```python
from build123d import *

# Parameters (mm, degrees)
SKETCH1_R           = 11.75
BOSS_EXTRUDE1_DEPTH = 60
CUT_EXTRUDE1_DEPTH  = 63.258533552
CUT_EXTRUDE2_DEPTH  = 64.608686514


with BuildPart() as part:
    # Sketch1 → Boss-Extrude1 (new body)
    with BuildSketch(Plane(origin=(0, 0, 0), x_dir=(0, 0, -1), z_dir=(1, 0, 0))):
        Circle(SKETCH1_R)
    extrude(amount=BOSS_EXTRUDE1_DEPTH)

    # Sketch2 → Cut-Extrude1 (cut, through all)
    with BuildSketch(Plane.ZY):
        with BuildLine():
            Line((5.8, 10.218732798), (5.8, -10.218732798))
            ThreePointArc((5.8, -10.218732798), (11.75, 0), (5.8, 10.218732798))
        make_face()
    extrude(amount=-CUT_EXTRUDE1_DEPTH, mode=Mode.SUBTRACT)

    # Sketch3 → Cut-Extrude2 (cut, through all)
    with BuildSketch(Plane.XY.offset(5.8)):
        with BuildLine():
            Line((0, 11.75), (60, 11.75))
            Line((60, 11.75), (60, -11.75))
            Line((60, -11.75), (44.282856857, -11.75))
            ThreePointArc((44.282856857, -11.75), (30, -5.75), (15.717143143, -11.75))
            Line((15.717143143, -11.75), (0, -11.75))
            Line((0, -11.75), (0, 11.75))
        make_face()
    extrude(amount=-CUT_EXTRUDE2_DEPTH, mode=Mode.SUBTRACT)


solid = part.part
```
Check sheet for the modelled part. Datum: model origin and axes. Units: mm. Give positions to 0.01 mm unless a question says otherwise; leave off trailing zeros. Order: outer loops, then holes, each group sorted by start corner. A loop starts at its lowest first (then second) coordinate and runs counter-clockwise, first axis right, second up. Notation, with made-up numbers: M 43,39 L 99,39 A21 ccw 99,71 Z; hole C -32,-16.75 d8. An arc over 180 degrees is marked long. Answer in a Markdown table with one row per item.
1) Cross-section at B-B, the plane z = 1.5. Enter the section's corners in (x, y), plus the area to 3 significant figures.
Filled sheet:
| item | result |
|---|---|
| outline | M 15.81,-11.65 L 44.19,-11.65 A20 ccw Z |
| area | 115 mm2 |
2) Gauge pin test, flat ends, axial feed: P1, Ø1, axis at x = 26, z = -6, coming from the +Y side; P2, Ø1.5, axis at x = 40.5, z = -5.5, coming from the -Y side; P3, Ø3, axis at y = -7.5, z = -3, coming from the -X side. Record the tip position at first contact, or that the pin passes through.
Filled sheet:
| item | result |
|---|---|
| P1 | stops at y = -6.06 |
| P2 | stops at y = -10.75 |
| P3 | stops at x = 19.07 |
3) Cross-section at D-D, the plane y = -11. Enter the section's corners in (x, z).
Filled sheet:
| item | result |
|---|---|
| outline | M 16.49,-4.13 L 43.51,-4.13 L 43.51,4.13 L 16.49,4.13 Z |
4) Thickness scan on L1, parallel to Z at x = 22.5, y = -9.75; L2, parallel to Z at x = 22.75, y = -7.5; L3, parallel to Y at x = 27.25, z = 4. Record the ranges inside material, lowest first. Write a range as [from, to].
Filled sheet:
| item | result |
|---|---|
| L1 | z = [-6.56, 5.8] |
| L2 | z = [-9.05, 5.8] |
| L3 | y = [-11.05, -5.94] |
5) Cross-section at C-C, the plane x = 35.25. Enter the section's corners in (y, z).
Filled sheet:
| item | result |
|---|---|
| outline | M -10.22,5.8 A11.75 ccw -6.45,-9.82 L -6.45,5.8 Z |
6) Cross-section at A-A, the plane y = -7.5. Enter the section's corners in (x, z), plus the area to 3 significant figures.
Filled sheet:
| item | result |
|---|---|
| outline | M 21.82,-9.05 L 38.18,-9.05 L 38.18,5.8 L 21.82,5.8 Z |
| area | 243 mm2 |
